Build history of the part. All positions in model axes, mm. Face numbers are marked on the shaded views. A direction names the side the tool comes from. Round coordinates to 2 decimals unless told otherwise and drop trailing zeros. Loops run counter-clockwise (first coordinate to the right, second up) from the corner with the lowest first, then second, coordinate; pieces in that order, holes last. Notation, with made-up numbers: (5, 12.5) -> (15, 12.5) arc R11 cw to (15, 19.5) -> close; hole circle Ø6 at (-34.75, -11). An arc over 180 degrees is marked (long way). Put each result on its own line as item: value. Start each with the question number.
Item 1: Cut at D-D, the plane x = 0. List the corners of the cut face in (y, z).
Item 2: Pull direction Z, two halves, no side cores. Call the marked faces 1, 2 and 3: +Z half, -Z half, draft (parallel to the pull), parting line (faces both ways), or undercut.
Item 3: Flat gauge pins, fed straight in: pin 1 Ø3.5 at (x, z) = (5.86, 69.14) entering from +Y; pin 2 Ø10 at (y, z) = (-2, 35.5) entering from +X; pin 3 Ø5 at (y, z) = (2, -20.5) entering from -X; pin 4 Ø6 at (y, z) = (-0.5, 65) entering from -X. Where does each tip first touch, or does it go through?
Item 4: Cut at C-C, the plane y = 3. Count the separate pieces of the cut face and the enclosed holes in it, plus the area to 3 significant figures.
Item 5: Drill centre lines: probe 1 along Z at (x, y) = (25, -2.75); probe 2 along Z at (x, y) = (28, -4.25); probe 3 along X at (y, z) = (-2.75, 30). Where is each one in solid material? Low to high. Write a range as [from, to].
Item 6: Tool access for the marked faces 4 and 5: list every direction of +Z, -Z, +X, -X, +Y, -Y with a clear straight run to the whole face (end or side of a thin tool).
Item 7: Cut at B-B, the plane x = 18. List the corners of the cut face in (y, z), plus the area to 3 significant figures.
Item 8: Cut at A-A, the plane z = -10. List the corners of the cut face in (x, y).
```python
from build123d import *

# Parameters (mm, degrees)
BOSS_EXTRUDE1_DEPTH = 10
SKETCH3_W           = 20
SKETCH3_H           = 20
BOSS_EXTRUDE2_DEPTH = 20
SKETCH2_R           = 2.1
CUT_EXTRUDE1_DEPTH  = 61.415229868


with BuildPart() as part:
    # Sketch1 → Boss-Extrude1 (new, symmetric)
    with BuildSketch(Plane(origin=(0, 0, 0), x_dir=(1, 0, 0), z_dir=(0, 1, 0))):
        with BuildLine():
            Line((10, 0), (10, 15))
            ThreePointArc((10, 15), (12.928932188, 22.071067812), (20, 25))
            Line((20, 25), (35, 25))
            Line((35, 25), (35, 45))
            Line((35, 45), (20, 45))
            ThreePointArc((20, 45), (-1.213203436, 36.213203436), (-10, 15))
            Line((-10, 15), (-10, 0))
            Line((-10, 0), (10, 0))
        make_face()
    extrude(amount=BOSS_EXTRUDE1_DEPTH, both=True)

    # Sketch3 → Boss-Extrude2 (add)
    with BuildSketch(Plane(origin=(0, 10, 0), x_dir=(1, 0, 0), z_dir=(0, 1, 0))):
        with Locations((0, -10)):
            Rectangle(SKETCH3_W, SKETCH3_H)
    extrude(amount=-BOSS_EXTRUDE2_DEPTH)

    # Sketch2 → Cut-Extrude1 (cut, through all)
    with BuildSketch(Plane(origin=(0, 10, 0), x_dir=(1, 0, 0), z_dir=(0, 1, 0))):
        with Locations(Location((5.857864376, 29.142135624, 0), (0, 0, 270))):
            Circle(SKETCH2_R)
        with Locations(Location((0, 10, 0), (0, 0, 270))):
            Circle(SKETCH2_R)
        with Locations(Location((25, 35, 0), (0, 0, 90))):
            Circle(SKETCH2_R)
        with Locations(Location((0, -10, 0), (0, 0, 270))):
            Circle(SKETCH2_R)
    extrude(amount=-CUT_EXTRUDE1_DEPTH, mode=Mode.SUBTRACT)

    # Mirror1: part across plane


with BuildPart() as part_1:
    add(part.part)
    add(part.part.mirror(Plane(origin=(10, -38.284271247, 20), x_dir=(1, 0, 0), z_dir=(0, 0, 1))))


solid = part_1.part
```
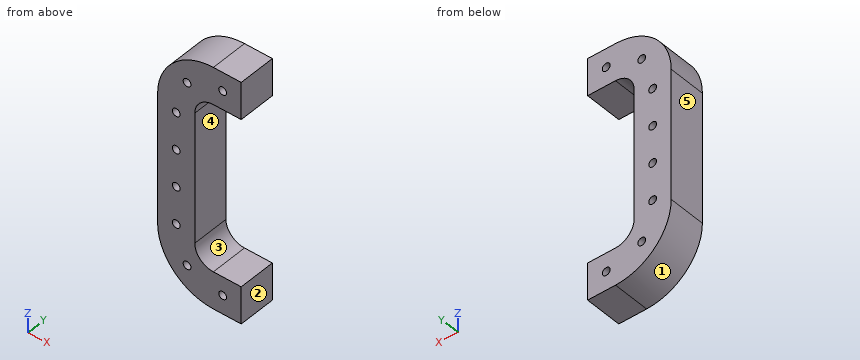
Reply:
1. outline: (-10, -37.36) -> (10, -37.36) -> (10, -12.1) -> (-10, -12.1) -> close; (-10, -7.9) -> (10, -7.9) -> (10, 7.9) -> (-10, 7.9) -> close; (-10, 12.1) -> (10, 12.1) -> (10, 27.9) -> (-10, 27.9) -> close; (-10, 32.1) -> (10, 32.1) -> (10, 47.9) -> (-10, 47.9) -> close; (-10, 52.1) -> (10, 52.1) -> (10, 77.36) -> (-10, 77.36) -> close
2. face 1: -Z half
2. face 2: draft
2. face 3: undercut
3. pin 1: passes through
3. pin 2: stops at x = 10
3. pin 3: stops at x = -9.85
3. pin 4: stops at x = -9.17
4. separate pieces: 1
4. enclosed holes: 8
4. area: 3,150 mm^2
5. probe 1: z = [-45, -37.1], [-32.9, -25], [65, 72.9], [77.1, 85]
5. probe 2: z = [-45, -25], [65, 85]
5. probe 3: x = [-10, -2.1], [2.1, 10]
6. face 4: +X, +Y, -Y
6. face 5: +Z, -Z, -X, +Y, -Y
7. outline: (-10, -44.93) -> (10, -44.93) -> (10, -24.8) -> (-10, -24.8) -> close; (-10, 64.8) -> (10, 64.8) -> (10, 84.93) -> (-10, 84.93) -> close
7. area: 805 mm^2
8. outline: (-10, -10) -> (-2.1, -10) -> (-2.1, 10) -> (-10, 10) -> close; (2.1, -10) -> (10, -10) -> (10, 10) -> (2.1, 10) -> close
